Geometry: final body of the model. Coordinates: model frame, mm. Coordinates: 2 decimals unless noted, no trailing zeros. Write each loop counter-clockwise with the first axis right and the second up, starting at its lowest first coordinate (ties: lowest second). Pieces come first, ordered by that corner, then holes. Notation, with made-up numbers: (-10.5, -17.5) - (-0.5, -17.5) arc R19 cw to (-0.5, -8.5) - close; hole circle Ø8 at (-15.5, 15.5). An arc over 180 degrees is marked (long way). Answer as a JSON object with one key per item and string values. Group by question number.
Item 1: First-contact query: pin 1 Ø1 at (x, z) = (1.5, 1) entering from -Y. Flat tip, straight axial feed; report the tip coordinate or a pass-through.
Item 2: Section A-A on x = 20.5. Return loops of the section in (y, z).
Item 3: Section C-C on y = 103.5. Return loops of the section in (x, z), and give its area (3 significant figures).
Item 4: Section D-D on x = -45.5. Return loops of the section in (y, z), and give its area (3 significant figures).
Item 5: Section B-B on z = 1.8. Return loops of the section in (x, y).
Item 6: Line query: line 1 along X through (y, z) = (122.5, 0.4); line 2 along Y through (x, z) = (30, 0.9); line 3 along X through (y, z) = (120, 1.5). Output: solid intervals per line, ascending. Write a range as from..to.
```python
from build123d import *

# Parameters (mm, degrees)
BOSS_EXTRUDE1_DEPTH = 3
BOSS_EXTRUDE2_DEPTH = 3


with BuildPart() as part:
    # Sketch7 → Boss-Extrude1 (new body)
    with BuildSketch(Plane.XY):
        Polygon((-78.549032868, 130.117059275), (38.237763696, 13.33026271), (38.237763696, -7.882940725), (17.02456026, -7.882940725), (-99.762236304, 108.903855839), (-99.762236304, 130.117059275), align=None)
    extrude(amount=BOSS_EXTRUDE1_DEPTH)

    # Sketch8 → Boss-Extrude2 (add)
    with BuildSketch(Plane.XY):
        Polygon((-78.549032868, -7.882940725), (38.237763696, 108.903855839), (38.237763696, 130.117059275), (17.02456026, 130.117059275), (-99.762236304, 13.33026271), (-99.762236304, -7.882940725), align=None)
    extrude(amount=BOSS_EXTRUDE2_DEPTH)


solid = part.part
```
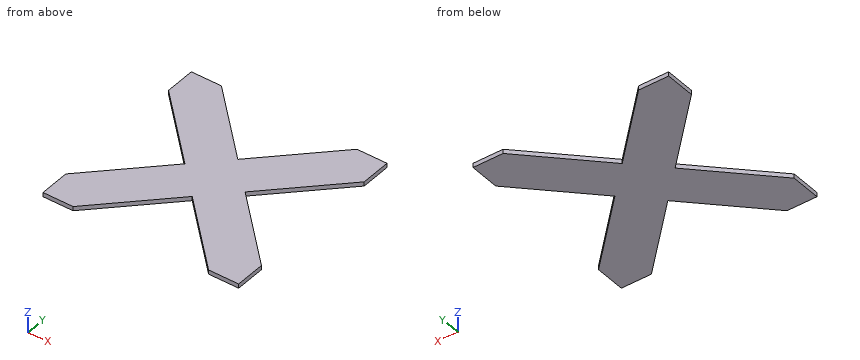
Checks:
{
 "1": {"pin 1": "y = 7.14"},
 "2": {"outline": "(-7.88, 0) - (31.07, 0) - (31.07, 3) - (-7.88, 3) - close; (91.17, 0) - (130.12, 0) - (130.12, 3) - (91.17, 3) - close"},
 "3": {"outline": "(-94.36, 0) - (-51.93, 0) - (-51.93, 3) - (-94.36, 3) - close; (-9.59, 0) - (32.83, 0) - (32.83, 3) - (-9.59, 3) - close", "area": "255 mm^2"},
 "4": {"outline": "(25.17, 0) - (97.07, 0) - (97.07, 3) - (25.17, 3) - close", "area": "216 mm^2"},
 "5": {"outline": "(-99.76, -7.88) - (-78.55, -7.88) - (-30.76, 39.9) - (17.02, -7.88) - (38.24, -7.88) - (38.24, 13.33) - (-9.55, 61.12) - (38.24, 108.9) - (38.24, 130.12) - (17.02, 130.12) - (-30.76, 82.33) - (-78.55, 130.12) - (-99.76, 130.12) - (-99.76, 108.9) - (-51.98, 61.12) - (-99.76, 13.33) - close"},
 "6": {"line 1": "-99.76..-70.93, 9.41..38.24", "line 2": "-7.88..21.57, 100.67..130.12", "line 3": "-99.76..-68.43, 6.91..38.24"}
}
